```python
from build123d import *

# Parameters (mm, degrees)
SKETCH_W        = 179
SKETCH_H        = 158
SKETCH_R        = 2.6
PAD_DEPTH       = 6
SKETCH001_W     = 5
SKETCH001_H     = 30
PAD001_DEPTH    = 30
SKETCH002_W     = 5
SKETCH002_H     = 35
PAD002_DEPTH    = 24
SKETCH003_R     = 2.6
POCKET_DEPTH    = 7
CHAMFER_SIZE    = 5
CHAMFER001_SIZE = 5
CHAMFER002_SIZE = 5
CHAMFER003_SIZE = 10
CHAMFER004_SIZE = 10
CHAMFER005_SIZE = 10


with BuildPart() as part:
    # Sketch → Pad (new body)
    with BuildSketch(Plane.XZ):
        with Locations((89.5, -79)):
            Rectangle(SKETCH_W, SKETCH_H)
        with Locations((89.5, -79)):
            Circle(SKETCH_R, mode=Mode.SUBTRACT)
        Polygon((16, -27.3), (16, -130.7), (78.185, -79), align=None, mode=Mode.SUBTRACT)
        Polygon((27.3, -142), (151.7, -142), (89.5, -90.315), align=None, mode=Mode.SUBTRACT)
        Polygon((163, -130.7), (163, -27.3), (100.815, -79), align=None, mode=Mode.SUBTRACT)
        Polygon((151.7, -16), (27.3, -16), (89.5, -67.685), align=None, mode=Mode.SUBTRACT)
    extrude(amount=-PAD_DEPTH)

    # Sketch001 (on Face3 of Pad) → Pad001 (join)
    with BuildSketch(Plane(origin=(179, 0, 0), x_dir=(0, 0, 1), z_dir=(1, 0, 0))):
        with Locations((-2.5, -15)):
            Rectangle(SKETCH001_W, SKETCH001_H)
    extrude(amount=PAD001_DEPTH)

    # Sketch002 (on Face3 of Pad001) → Pad002 (join)
    with BuildSketch(Plane(origin=(0, 6, 0), x_dir=(1, 0, 0), z_dir=(0, 1, 0))):
        with Locations((176.5, 17.5)):
            Rectangle(SKETCH002_W, SKETCH002_H)
    extrude(amount=PAD002_DEPTH)

    # Sketch003 (on Face22 of Pad002) → Pocket (cut)
    with BuildSketch(Plane(origin=(0, 0, 0), x_dir=(-1, 0, 0), z_dir=(0, 0, 1))):
        with Locations((-194, -15)):
            Circle(SKETCH003_R)
    extrude(amount=-POCKET_DEPTH, mode=Mode.SUBTRACT)

    # Chamfer
    chamfer_edges = [part.edges().sort_by_distance(p)[0] for p in [
        (209, 30, -2.5),
        (209, 0, -2.5),
    ]]
    chamfer(chamfer_edges, length=CHAMFER_SIZE)

    # Chamfer001
    chamfer001_edges = [part.edges().sort_by_distance(p)[0] for p in [
        (176.5, 30, -35),
    ]]
    chamfer(chamfer001_edges, length=CHAMFER001_SIZE)

    # Chamfer002
    chamfer002_edges = [part.edges().sort_by_distance(p)[0] for p in [
        (176.5, 6, -35),
    ]]
    chamfer(chamfer002_edges, length=CHAMFER002_SIZE)

    # Chamfer003
    chamfer003_edges = [part.edges().sort_by_distance(p)[0] for p in [
        (179, 3, -158),
    ]]
    chamfer(chamfer003_edges, length=CHAMFER003_SIZE)

    # Chamfer004
    chamfer004_edges = [part.edges().sort_by_distance(p)[0] for p in [
        (0, 3, -158),
    ]]
    chamfer(chamfer004_edges, length=CHAMFER004_SIZE)

    # Chamfer005
    chamfer005_edges = [part.edges().sort_by_distance(p)[0] for p in [
        (0, 3, 0),
    ]]
    chamfer(chamfer005_edges, length=CHAMFER005_SIZE)


solid = part.part
```
Work out the finished part from the listing and answer in its coordinate system (mm). A direction names the side the tool comes from. Coordinates: 2 decimals unless noted, no trailing zeros. Loops run counter-clockwise (first coordinate to the right, second up) from the corner with the lowest first, then second, coordinate; pieces in that order, holes last. Notation, with made-up numbers: (50, 69) -> (98, 69) arc R29 cw to (98, 94) -> close; hole circle Ø4 at (18, 41.25). An arc over 180 degrees is marked (long way). Answer as CSV lines item,"result".
Q1. The part is cut by section C-C on z = -44. Write down the section's boundary in (x, y), and give its area (3 significant figures).
Findings:
outline,"(0, 0) -> (16, 0) -> (16, 6) -> (0, 6) -> close; (36.09, 0) -> (61, 0) -> (61, 6) -> (36.09, 6) -> close; (118, 0) -> (142.91, 0) -> (142.91, 6) -> (118, 6) -> close; (163, 0) -> (179, 0) -> (179, 6) -> (163, 6) -> close"
area,"491 mm²"
Q2. For a pull along X with two mould halves and no side action, classify faces 1 (the face through (121.035, 2.958, -116.519)), 2 (the face through (209, 15, -3)), 3 (the face through (0, 3, -80)) as +X half, -X half, draft (parallel to the pull), parting line (faces both ways), or undercut.
Findings:
face 1,"undercut"
face 2,"+X half"
face 3,"-X half"
Q3. A tool of negligible diameter and unlimited length cuts with its end or side. For faces 4 (the face through (16, 3, -78)), 5 (the face through (206, 2, -3)), 6 (the face through (190, 15, -5)), 7 (the face through (174, 18, -20)), 8 (the face through (178, 30, -10)), from which of +Z, -Z, +X, -X, +Y, -Y can it reach the whole face along a straight path? Write none if from no direction.
Findings:
face 4,"+Y, -Y"
face 5,"+Z, -Z, +X, -Y"
face 6,"-Z, +X, +Y, -Y"
face 7,"+Z, -Z, -X, +Y"
face 8,"+Z, -Z, +X, -X, +Y"
Q4. Each of these flat-tipped pins is pushed along its axis until it touches: pin 1 (1 mm diameter, centred on x = 143, z = -134.5, fed in from +Y); pin 2 (2 mm diameter, centred on x = 34.5, y = 8, fed in from -Z); pin 3 (12 mm diameter, centred on y = 21, z = -24.5, fed in from -X); pin 4 (2.5 mm diameter, centred on x = 177.5, y = 16, fed in from -Z). Where does it stop, or does it pass through?
Findings:
pin 1,"stops at y = 6"
pin 2,"passes through"
pin 3,"stops at x = 174"
pin 4,"stops at z = -35"
Q5. Find the intervals of material crossed by probe 1 along Y at (x, z) = (194, -3.1); probe 2 along X at (y, z) = (3, -92.5); probe 3 along X at (y, z) = (15, -2), in increasing order.
Findings:
probe 1,"y = 0 to 12.4, 17.6 to 30"
probe 2,"x = 0 to 16, 61.95 to 86.87, 92.13 to 117.05, 163 to 179"
probe 3,"x = 174 to 191.4, 196.6 to 209"
Q6. The part is cut by section A-A on y = 15. Write down the section's boundary in (x, z).
Findings:
outline,"(174, -35) -> (179, -35) -> (179, -5) -> (191.4, -5) -> (191.4, 0) -> (174, 0) -> close; (196.6, -5) -> (209, -5) -> (209, 0) -> (196.6, 0) -> close"
Q7. The part is cut by section B-B on x = 194. Write down the section's boundary in (y, z), and give its area (3 significant figures).
Findings:
outline,"(0, -5) -> (12.4, -5) -> (12.4, 0) -> (0, 0) -> close; (17.6, -5) -> (30, -5) -> (30, 0) -> (17.6, 0) -> close"
area,"124 mm²"
Q8. The part is cut by section D-D on x = 55. Write down the section's boundary in (y, z).
Findings:
outline,"(0, -158) -> (6, -158) -> (6, -142) -> (0, -142) -> close; (0, -118.98) -> (6, -118.98) -> (6, -98.28) -> (0, -98.28) -> close; (0, -59.72) -> (6, -59.72) -> (6, -39.02) -> (0, -39.02) -> close; (0, -16) -> (6, -16) -> (6, 0) -> (0, 0) -> close"
